```python
from build123d import *

# Parameters (mm, degrees)
SKETCH2_R           = 1
SKETCH2_R_2         = 2
BOSS_EXTRUDE2_DEPTH = 5


with BuildPart() as part:
    # Sketch2 → Boss-Extrude2 (new body)
    with BuildSketch(Plane.XY):
        with BuildLine():
            Line((10.773856573, 0), (-10.773856573, 0))
            ThreePointArc((-10.773856573, 0), (-12.807539789, -0.432272712), (-14.489580701, -1.654346968))
            Line((-14.489580701, -1.654346968), (-32.85230533, -22.048218747))
            ThreePointArc((-32.85230533, -22.048218747), (-33.804483335, -23.602032031), (-34.136581202, -25.393871779))
            Line((-34.136581202, -25.393871779), (-34.136581202, -27.926924356))
            ThreePointArc((-34.136581202, -27.926924356), (-34.681548581, -30.196876855), (-36.197654941, -31.972009328))
            Line((-36.197654941, -31.972009328), (-47.938926261, -40.502542276))
            Line((-47.938926261, -40.502542276), (-49.271172991, -33.33925419))
            ThreePointArc((-49.271172991, -33.33925419), (-50.646968461, -29.828950283), (-53.224733986, -27.077555801))
            Line((-53.224733986, -27.077555801), (-69.848063434, -15))
            Line((-69.848063434, -15), (-69.848063434, -97.913369077))
            ThreePointArc((-69.848063434, -97.913369077), (-68.307820915, -103.245582818), (-64.161562759, -106.935216093))
            Line((-64.161562759, -106.935216093), (-50, -113.7061014))
            ThreePointArc((-50, -113.7061014), (-49.840547901, -114.95873703), (-49.372361591, -116.131478508))
            Line((-49.372361591, -116.131478508), (-38.744938669, -135.290122192))
            ThreePointArc((-38.744938669, -135.290122192), (-36.909614174, -137.173276478), (-34.372577077, -137.864745084))
            Line((-34.372577077, -137.864745084), (-29.364406032, -137.864745084))
            ThreePointArc((-29.364406032, -137.864745084), (-27.094453533, -138.409712463), (-25.31932106, -139.925818823))
            Line((-25.31932106, -139.925818823), (-19.497457724, -147.938926261))
            ThreePointArc((-19.497457724, -147.938926261), (-17.722325251, -149.455032621), (-15.452372753, -150))
            Line((-15.452372753, -150), (15.452372753, -150))
            ThreePointArc((15.452372753, -150), (17.722325251, -149.455032621), (19.497457724, -147.938926261))
            Line((19.497457724, -147.938926261), (25.31932106, -139.925818823))
            ThreePointArc((25.31932106, -139.925818823), (27.094453533, -138.409712463), (29.364406032, -137.864745084))
            Line((29.364406032, -137.864745084), (34.372577077, -137.864745084))
            ThreePointArc((34.372577077, -137.864745084), (36.909614174, -137.173276478), (38.744938669, -135.290122192))
            Line((38.744938669, -135.290122192), (49.372361591, -116.131478508))
            ThreePointArc((49.372361591, -116.131478508), (49.840547901, -114.95873703), (50, -113.7061014))
            Line((50, -113.7061014), (64.161562759, -106.935216093))
            ThreePointArc((64.161562759, -106.935216093), (68.307820915, -103.245582818), (69.848063434, -97.913369077))
            Line((69.848063434, -97.913369077), (69.848063434, -15))
            Line((69.848063434, -15), (53.224733986, -27.077555801))
            ThreePointArc((53.224733986, -27.077555801), (50.646968461, -29.828950283), (49.271172991, -33.33925419))
            Line((49.271172991, -33.33925419), (47.938926261, -40.502542276))
            Line((47.938926261, -40.502542276), (36.197654941, -31.972009328))
            ThreePointArc((36.197654941, -31.972009328), (34.681548581, -30.196876855), (34.136581202, -27.926924356))
            Line((34.136581202, -27.926924356), (34.136581202, -25.393871779))
            ThreePointArc((34.136581202, -25.393871779), (33.804483335, -23.602032031), (32.85230533, -22.048218747))
            Line((32.85230533, -22.048218747), (14.489580701, -1.654346968))
            ThreePointArc((14.489580701, -1.654346968), (12.807539789, -0.432272712), (10.773856573, 0))
        make_face()
        with Locations((0, -5)):
            Circle(SKETCH2_R, mode=Mode.SUBTRACT)
        with Locations((0, -145)):
            Circle(SKETCH2_R_2, mode=Mode.SUBTRACT)
        with Locations((0, -105)):
            Circle(SKETCH2_R_2, mode=Mode.SUBTRACT)
        with Locations((-12, -50.308044585)):
            Circle(SKETCH2_R_2, mode=Mode.SUBTRACT)
        with Locations((12, -50.308044585)):
            Circle(SKETCH2_R_2, mode=Mode.SUBTRACT)
        with Locations((12, -85.308044585)):
            Circle(SKETCH2_R_2, mode=Mode.SUBTRACT)
        with Locations((-12, -85.308044585)):
            Circle(SKETCH2_R_2, mode=Mode.SUBTRACT)
        with Locations((-34.372577077, -132.864745084)):
            Circle(SKETCH2_R_2, mode=Mode.SUBTRACT)
        with Locations((34.372577077, -132.864745084)):
            Circle(SKETCH2_R_2, mode=Mode.SUBTRACT)
        with Locations((-45, -44.547627247)):
            Circle(SKETCH2_R_2, mode=Mode.SUBTRACT)
        with Locations((45, -44.547627247)):
            Circle(SKETCH2_R_2, mode=Mode.SUBTRACT)
        with Locations((-65.664848414, -23.474551604)):
            Circle(SKETCH2_R_2, mode=Mode.SUBTRACT)
        with Locations((65.664848414, -23.474551604)):
            Circle(SKETCH2_R_2, mode=Mode.SUBTRACT)
        with BuildLine():
            Line((-12.660728973, -13.073490301), (-26.043341101, -27.93638681))
            ThreePointArc((-26.043341101, -27.93638681), (-28.867891964, -28.084415248), (-29.015920402, -25.259864385))
            Line((-29.015920402, -25.259864385), (-15.633308275, -10.396967875))
            ThreePointArc((-15.633308275, -10.396967875), (-12.808757412, -10.248939437), (-12.660728973, -13.073490301))
        make_face(mode=Mode.SUBTRACT)
        with BuildLine():
            Line((14.147018624, -37.43638681), (19.147018624, -37.43638681))
            ThreePointArc((19.147018624, -37.43638681), (20.458982346, -36.663539609), (20.41901608, -35.1413884))
            Line((20.41901608, -35.1413884), (15.41901608, -27.1413884))
            ThreePointArc((15.41901608, -27.1413884), (13.733494855, -26.494513691), (12.647018624, -27.93638681))
            Line((12.647018624, -27.93638681), (12.647018624, -35.93638681))
            ThreePointArc((12.647018624, -35.93638681), (13.086358453, -36.997046982), (14.147018624, -37.43638681))
        make_face(mode=Mode.SUBTRACT)
        with BuildLine():
            Line((-14.147018624, -37.43638681), (-19.147018624, -37.43638681))
            ThreePointArc((-19.147018624, -37.43638681), (-20.458982346, -36.663539609), (-20.41901608, -35.1413884))
            Line((-20.41901608, -35.1413884), (-15.41901608, -27.1413884))
            ThreePointArc((-15.41901608, -27.1413884), (-13.733494855, -26.494513691), (-12.647018624, -27.93638681))
            Line((-12.647018624, -27.93638681), (-12.647018624, -35.93638681))
            ThreePointArc((-12.647018624, -35.93638681), (-13.086358453, -36.997046982), (-14.147018624, -37.43638681))
        make_face(mode=Mode.SUBTRACT)
        with BuildLine():
            Line((12.660728973, -13.073490301), (26.043341101, -27.93638681))
            ThreePointArc((26.043341101, -27.93638681), (28.867891964, -28.084415248), (29.015920402, -25.259864385))
            Line((29.015920402, -25.259864385), (15.633308275, -10.396967875))
            ThreePointArc((15.633308275, -10.396967875), (12.808757412, -10.248939437), (12.660728973, -13.073490301))
        make_face(mode=Mode.SUBTRACT)
        with BuildLine():
            Line((1.5, -15), (1.5, -30))
            ThreePointArc((1.5, -30), (0, -31.5), (-1.5, -30))
            Line((-1.5, -30), (-1.5, -15))
            ThreePointArc((-1.5, -15), (0, -13.5), (1.5, -15))
        make_face(mode=Mode.SUBTRACT)
        with BuildLine():
            Line((-65.664848414, -46.221025879), (-52.228109947, -55.148662815))
            ThreePointArc((-52.228109947, -55.148662815), (-51.808846465, -57.228138261), (-53.888321911, -57.647401744))
            Line((-53.888321911, -57.647401744), (-67.325060378, -48.719764808))
            ThreePointArc((-67.325060378, -48.719764808), (-67.744323861, -46.640289361), (-65.664848414, -46.221025879))
        make_face(mode=Mode.SUBTRACT)
        with BuildLine():
            Line((-65.664848414, -59.427687694), (-52.228109947, -68.35532463))
            ThreePointArc((-52.228109947, -68.35532463), (-51.808846465, -70.434800076), (-53.888321911, -70.854063559))
            Line((-53.888321911, -70.854063559), (-67.325060378, -61.926426623))
            ThreePointArc((-67.325060378, -61.926426623), (-67.744323861, -59.846951176), (-65.664848414, -59.427687694))
        make_face(mode=Mode.SUBTRACT)
        with BuildLine():
            Line((-65.664848414, -72.634349509), (-52.228109947, -81.561986445))
            ThreePointArc((-52.228109947, -81.561986445), (-51.808846465, -83.641461891), (-53.888321911, -84.060725374))
            Line((-53.888321911, -84.060725374), (-67.325060378, -75.133088438))
            ThreePointArc((-67.325060378, -75.133088438), (-67.744323861, -73.053612992), (-65.664848414, -72.634349509))
        make_face(mode=Mode.SUBTRACT)
        with BuildLine():
            Line((-50.329634754, -108.179131466), (-60.893208182, -102.243321386))
            ThreePointArc((-60.893208182, -102.243321386), (-64.625452121, -98.575764145), (-65.994483169, -93.525380502))
            Line((-65.994483169, -93.525380502), (-65.994483169, -90.405290348))
            Line((-65.994483169, -90.405290348), (-55.430909741, -96.341100429))
            ThreePointArc((-55.430909741, -96.341100429), (-51.698665801, -100.00865767), (-50.329634754, -105.059041312))
            Line((-50.329634754, -105.059041312), (-50.329634754, -108.179131466))
        make_face(mode=Mode.SUBTRACT)
        with BuildLine():
            Line((65.664848414, -46.221025879), (52.228109947, -55.148662815))
            ThreePointArc((52.228109947, -55.148662815), (51.808846465, -57.228138261), (53.888321911, -57.647401744))
            Line((53.888321911, -57.647401744), (67.325060378, -48.719764808))
            ThreePointArc((67.325060378, -48.719764808), (67.744323861, -46.640289361), (65.664848414, -46.221025879))
        make_face(mode=Mode.SUBTRACT)
        with BuildLine():
            Line((65.664848414, -59.427687694), (52.228109947, -68.35532463))
            ThreePointArc((52.228109947, -68.35532463), (51.808846465, -70.434800076), (53.888321911, -70.854063559))
            Line((53.888321911, -70.854063559), (67.325060378, -61.926426623))
            ThreePointArc((67.325060378, -61.926426623), (67.744323861, -59.846951176), (65.664848414, -59.427687694))
        make_face(mode=Mode.SUBTRACT)
        with BuildLine():
            Line((65.664848414, -72.634349509), (52.228109947, -81.561986445))
            ThreePointArc((52.228109947, -81.561986445), (51.808846465, -83.641461891), (53.888321911, -84.060725374))
            Line((53.888321911, -84.060725374), (67.325060378, -75.133088438))
            ThreePointArc((67.325060378, -75.133088438), (67.744323861, -73.053612992), (65.664848414, -72.634349509))
        make_face(mode=Mode.SUBTRACT)
        with BuildLine():
            Line((65.994483169, -90.405290348), (55.430909741, -96.341100429))
            ThreePointArc((55.430909741, -96.341100429), (51.698665801, -100.00865767), (50.329634754, -105.059041312))
            Line((50.329634754, -105.059041312), (50.329634754, -108.179131466))
            Line((50.329634754, -108.179131466), (60.893208182, -102.243321386))
            ThreePointArc((60.893208182, -102.243321386), (64.625452121, -98.575764145), (65.994483169, -93.525380502))
            Line((65.994483169, -93.525380502), (65.994483169, -90.405290348))
        make_face(mode=Mode.SUBTRACT)
    extrude(amount=BOSS_EXTRUDE2_DEPTH)


solid = part.part
```
For this review, take the finished solid that the model builds, in its own axes (mm). A direction names the side the tool comes from. Coordinates: 2 decimals unless noted, no trailing zeros. Write each loop counter-clockwise with the first axis right and the second up, starting at its lowest first coordinate (ties: lowest second). Pieces come first, ordered by that corner, then holes. Notation, with made-up numbers: (-34, 68) - (17, 68) arc R22 ccw to (17, 99) - close; hole circle Ø5 at (65.25, -18.5). An arc over 180 degrees is marked (long way). Put each result on its own line as item: value.
1. Wall thickness on probe 1 along Y at (x, z) = (0, 1.15); probe 2 along X at (y, z) = (-62.5, 1.3); probe 3 along X at (y, z) = (-47.5, 3.25): over which ranges is each line inside the solid? List them lowest first.
Values found:
probe 1: -150 to -147, -143 to -107, -103 to -31.5, -13.5 to -6, -4 to 0
probe 2: -69.85 to -66.46, -61.04 to 61.04, 66.46 to 69.85
probe 3: -69.85 to -67.99, -63.74 to 63.74, 67.99 to 69.85
2. Add section C-C, the plane z = 1.95. Count the separate pieces of the cut face and the enclosed holes in it, then the cut area to 3 significant figures.
Values found:
separate pieces: 1
enclosed holes: 26
area: 14,700 mm²
3. Add section A-A, the plane y = -78. Give the boundary of the cut face in (x, z), then the cut area to 3 significant figures.
Values found:
outline: (-69.85, 0) - (-63.01, 0) - (-63.01, 5) - (-69.85, 5) - close; (-57.59, 0) - (57.59, 0) - (57.59, 5) - (-57.59, 5) - close; (63.01, 0) - (69.85, 0) - (69.85, 5) - (63.01, 5) - close
area: 644 mm²
4. For pin 1 (2 mm diameter, centred on x = -22.5, z = 4.5, fed in from -Y); pin 2 (1.5 mm diameter, centred on x = 32, z = 3.5, fed in from -Y); pin 3 (1.5 mm diameter, centred on x = -14, z = 0.5, fed in from +Y), all flat-tipped, find the tip position at first contact; note any pin that passes through.
Values found:
pin 1: y = -145.18
pin 2: y = -137.86
pin 3: y = -0.66
5. Mouldability with a two-part tool opening along Y and no side actions: class faces 1 (the cylindrical face through (33.814, -23.626, 2.465)), 2 (the flat face through (1.5, -22, 2)), 3 (the cylindrical face through (-27.124, -138.395, 2.465)) as released by +Y, released by -Y, zero draft, split by the parting line, or undercut.
Values found:
face 1: released by +Y
face 2: undercut
face 3: released by -Y
6. Add section D-D, the plane y = -120.5. Give the boundary of the cut face in (x, z), then the cut area to 3 significant figures.
Values found:
outline: (-46.95, 0) - (46.95, 0) - (46.95, 5) - (-46.95, 5) - close
area: 469 mm²
7. Machinability: for faces 4 (the flat face through (-1, -74, 0)), 5 (the flat face through (32, -137.865, 2)), 6 (the cylindrical face through (34.7, -30.23, 2.46)), 7 (the cylindrical face through (51.74, -99.94, 2.46)), which of the approach directions +Z, -Z, +X, -X, +Y, -Y give a long, thin tool a straight path to every point of the face, cutting with its end or side? Answer none if there is none.
Values found:
face 4: -Z, +X, -X, +Y, -Y
face 5: +Z, -Z, +X, -Y
face 6: +Z, -Z, +Y
face 7: +Z, -Z
8. Add section B-B, the plane x = -45. Give the boundary of the cut face in (y, z).
Values found:
outline: (-124.01, 0) - (-46.55, 0) - (-46.55, 5) - (-124.01, 5) - close; (-42.55, 0) - (-38.37, 0) - (-38.37, 5) - (-42.55, 5) - close
